Design review of the part shown in the three views and the two pictorial views. Dimensions are in mm from the part's minimum x, y and z. A direction names the side the tool comes from. Give positions to 0.01 mm unless a question says otherwise; leave off trailing zeros. Order: outer loops, then holes, each group sorted by start corner. A loop starts at its lowest first (then second) coordinate and runs counter-clockwise, first axis right, second up. Notation, with made-up numbers: (40.5, 44) -> (79.5, 44) arc R23 cw to (79.5, 71) -> close; hole circle Ø3 at (-18, 8.25). An arc over 180 degrees is marked (long way). Use one line per item in the form item = value.
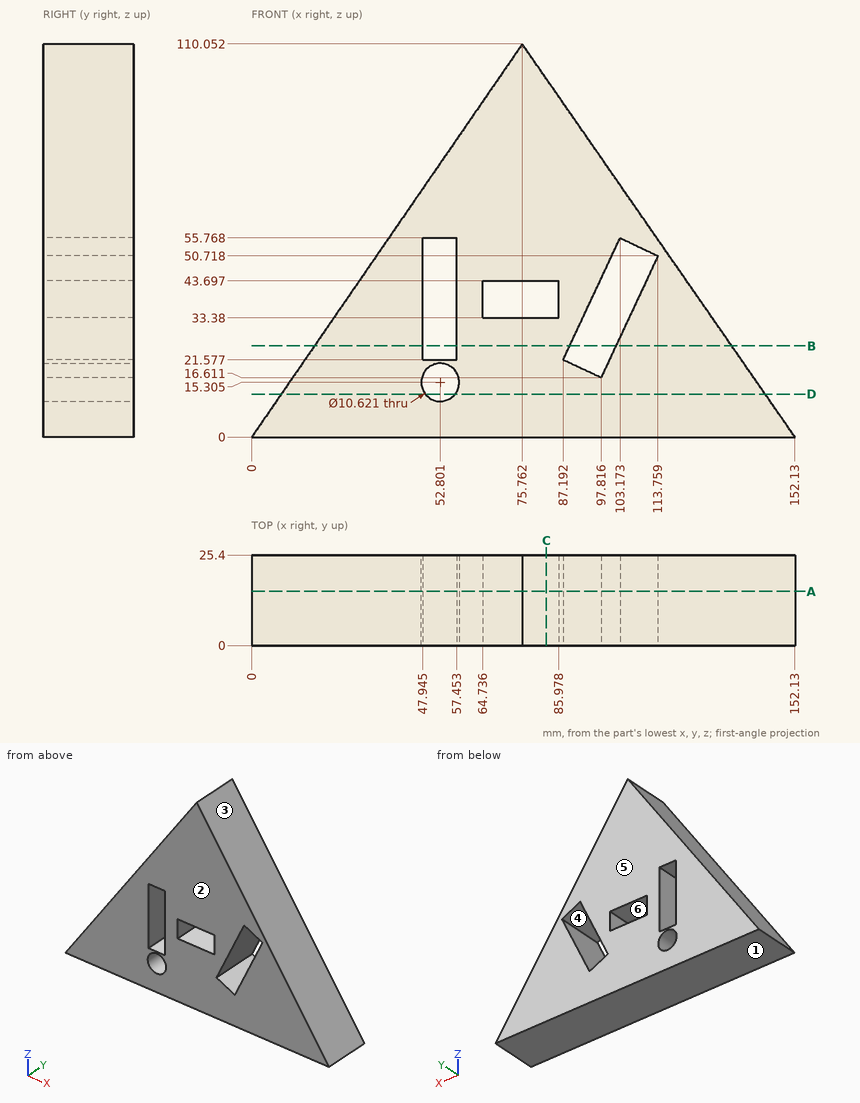
1. Add section A-A on y = 15.25. Give the boundary of the cut face in (x, z) (1 decimal), then the cut area to 3 significant figures.
Values:
outline = (0, 0) -> (152.1, 0) -> (75.8, 110.1) -> close; hole circle Ø10.6 at (52.8, 15.3); hole (47.9, 21.6) -> (57.5, 21.6) -> (57.5, 55.8) -> (47.9, 55.8) -> close; hole (64.7, 33.4) -> (86, 33.4) -> (86, 43.7) -> (64.7, 43.7) -> close; hole (87.2, 21.6) -> (97.8, 16.6) -> (113.8, 50.7) -> (103.2, 55.8) -> close
area = 7,300 mm^2
2. Add section B-B on z = 25.5. Give the boundary of the cut face in (x, y) (1 decimal), then the cut area to 3 significant figures.
Values:
outline = (17.6, 0) -> (47.9, 0) -> (47.9, 25.4) -> (17.6, 25.4) -> close; (57.5, 0) -> (89, 0) -> (89, 25.4) -> (57.5, 25.4) -> close; (102, 0) -> (134.4, 0) -> (134.4, 25.4) -> (102, 25.4) -> close
area = 2,400 mm^2
3. For L1, parallel to X at y = 18.75, z = 38 (1 decimal); L2, parallel to X at y = 22, z = 24 (1 decimal); L3, parallel to X at y = 10.25, z = 28.5 (1 decimal), list the stretches that pass through material, from the lowest coordinate up.
Values:
L1 = 26.2 to 47.9, 57.5 to 64.7, 86 to 94.9, 107.8 to 125.8
L2 = 16.5 to 47.9, 57.5 to 88.3, 101.3 to 135.5
L3 = 19.6 to 47.9, 57.5 to 90.4, 103.4 to 132.4
4. Add section D-D on z = 12. Give the boundary of the cut face in (x, y) (1 decimal).
Values:
outline = (8.3, 0) -> (48.6, 0) -> (48.6, 25.4) -> (8.3, 25.4) -> close; (57, 0) -> (143.8, 0) -> (143.8, 25.4) -> (57, 25.4) -> close
5. The part is to be moulded in two halves that separate along Z. For the marked faces 1, 2, 3 and 4, say which applies: +Z half, -Z half, draft (parallel to the pull), parting line (faces both ways), or undercut.
Values:
face_1 = -Z half
face_2 = draft
face_3 = +Z half
face_4 = undercut
6. Add section C-C on x = 82.5. Give the boundary of the cut face in (y, z).
Values:
outline = (0, 0) -> (25.4, 0) -> (25.4, 33.38) -> (0, 33.38) -> close; (0, 43.7) -> (25.4, 43.7) -> (25.4, 100.34) -> (0, 100.34) -> close
7. Tool access review of the marked faces 5 and 6: name each direction out of +Z, -Z, +X, -X, +Y, -Y from which nothing blocks a thin tool from reaching the whole face with its end or side.
Values:
face_5 = +Z, -Z, +X, -X, +Y
face_6 = +Y, -Y
8. For pin 1 Ø7.5 at (x, y) = (54.5, 10.5) entering from +Z (1 decimal); pin 2 Ø5 at (y, z) = (7, 37) entering from +X; pin 3 Ø1.5 at (y, z) = (2.5, 94.5) entering from +X (1 decimal); pin 4 Ø10 at (x, z) = (46, 58.5) entering from -Y, all flat-tipped, find the tip position at first contact; note any pin that passes through.
Values:
pin_1 = 84.6
pin_2 = 128.19
pin_3 = 87.1
pin_4 = 0
